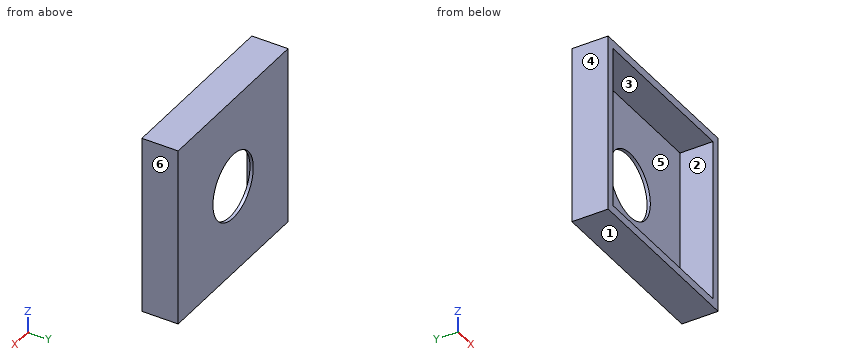
from build123d import *

# Parameters (mm, degrees)
F4_W     = 109
F4_H     = 109
F5_DEPTH = 22
F6_T     = -5
F7_DEPTH = 3
F9_D     = 40


with BuildPart() as f5:
    # F4 (on Front) → F5 (new body)
    with BuildSketch(Plane.XZ):
        Rectangle(F4_W, F4_H)
    extrude(amount=F5_DEPTH)

    # F6
    f6_openings = [f5.faces().sort_by_distance(p)[0] for p in [
        (0, -22, 0),
    ]]
    offset(amount=F6_T, openings=f6_openings)

    # F7 (cut): a face of the model
    f7_faces = [f5.faces().sort_by_distance(p)[0] for p in [
        (0, -5, 0),
    ]]
    extrude(f7_faces, amount=-F7_DEPTH, mode=Mode.SUBTRACT)

    # F9 (through all)
    with Locations(Plane(origin=(0, 0, 0), x_dir=(-1, 0, 0), z_dir=(0, 1, 0))):
        with Locations((0, 0)):
            Hole(F9_D / 2)


solid = f5.part
Read the model definition and answer for the solid it produces. Units are mm, in the model's axes. Face numbers are marked on the shaded views. A direction names the side the tool comes from. Round coordinates to 2 decimals unless told otherwise and drop trailing zeros. Write each loop counter-clockwise with the first axis right and the second up, starting at its lowest first coordinate (ties: lowest second). Pieces come first, ordered by that corner, then holes.
1. Determine the mould class of the marked faces 1, 2, 3 and 4 for opening direction Z: pulls with the +Z half, pulls with the -Z half, needs draft (parallel to the pull), parting line crosses it, or undercut.
2. The part is cut by section C-C, the plane x = -39.5. Determine the outline of the cut face in (y, z).
3. Which of the six approach directions +Z, -Z, +X, -X, +Y, -Y give full straight-line access (tool end or side, diameter ignored) to the marked faces 5 and 6?
4. The part is cut by section A-A, the plane x = 0. Determine the outline of the cut face in (y, z).
5. The part is cut by section B-B, the plane z = 0. Determine the outline of the cut face in (x, y), then the cut area to 3 significant figures.
6. The part is cut by section D-D, the plane y = -16. Determine the outline of the cut face in (x, z).
7. Straight lines are drawn through the part: L1, parallel to Z at x = -10, y = -9; L2, parallel to Z at x = 0, y = -1.3. For each, find the intervals that lie inside material, in ascending order.
Values:
1. face 1: pulls with the -Z half
1. face 2: undercut
1. face 3: undercut
1. face 4: needs draft
2. outline: (-22, -54.5) - (0, -54.5) - (0, 54.5) - (-22, 54.5) - (-22, 49.5) - (-2, 49.5) - (-2, -49.5) - (-22, -49.5) - close
3. face 5: -Y
3. face 6: +Z, -Z, +X, +Y, -Y
4. outline: (-22, -54.5) - (0, -54.5) - (0, -20) - (-2, -20) - (-2, -49.5) - (-22, -49.5) - close; (-22, 49.5) - (-2, 49.5) - (-2, 20) - (0, 20) - (0, 54.5) - (-22, 54.5) - close
5. outline: (-54.5, -22) - (-49.5, -22) - (-49.5, -2) - (-20, -2) - (-20, 0) - (-54.5, 0) - close; (20, -2) - (49.5, -2) - (49.5, -22) - (54.5, -22) - (54.5, 0) - (20, 0) - close
5. area: 338 mm2
6. outline: (-54.5, -54.5) - (54.5, -54.5) - (54.5, 54.5) - (-54.5, 54.5) - close; hole (-49.5, -49.5) - (49.5, -49.5) - (49.5, 49.5) - (-49.5, 49.5) - close
7. L1: z = -54.5 to -49.5, 49.5 to 54.5
7. L2: z = -54.5 to -20, 20 to 54.5
